Build history of the part. All positions in model axes, mm. A direction names the side the tool comes from. Round coordinates to 2 decimals unless told otherwise and drop trailing zeros. Write each loop counter-clockwise with the first axis right and the second up, starting at its lowest first coordinate (ties: lowest second). Pieces come first, ordered by that corner, then holes. Notation, with made-up numbers: M 5,21 L 23,21 A4 ccw 23,26 Z; hole C 12,-10 d10. An arc over 180 degrees is marked long. Write item = value, one per line. Start each with the question number.
Q1. Band-saw the part on A-A on x = 0. Write the cut outline in (y, z).
Q2. Drop flat-ended pins along their axis: P1, Ø1.5, axis at y = 0, z = 2.5, coming from the +X side; P2, Ø1, axis at y = -2.5, z = -1.5, coming from the +X side; P3, Ø1.5, axis at x = -0.5, y = -5.5, coming from the +Z side. Give the stop position or say it passes through.
Q3. Tool access for faces 1 (the flat face through (4.96, 2.81, -1.65)), 2 (the cylindrical face through (0, 2, 7)), 3 (the flat face through (0, 5.7, -2)), 4 (the flat face through (0, -5.7, -2)): list every direction of +Z, -Z, +X, -X, +Y, -Y with a clear straight run to the whole face (end or side of a thin tool).
Q4. Band-saw the part on B-B on y = 4. Write the cut outline in (x, z), plus the area to 3 significant figures.
Q5. Probe L1, parallel to Z at x = 5, y = 2.25; L2, parallel to Y at x = 1.5, z = -0.75; L3, parallel to X at y = -0.75, z = 0.5. List the from-to ranges inside material, lowest first.
Q6. Band-saw the part on C-C on z = 0.5. Write the cut outline in (x, y), plus the area to 3 significant figures.
Q7. Band-saw the part on D-D on x = 2.75. Write the cut outline in (y, z), plus the area to 3 significant figures.
```python
from build123d import *

# Parameters (mm, degrees)
SKETCH1_R           = 7.5
SKETCH1_R_2         = 5.6
BOSS_EXTRUDE1_DEPTH = 1
BOSS_EXTRUDE2_DEPTH = 3.35
BOSS_EXTRUDE3_START = 1
SKETCH1_4_R         = 5.6
BOSS_EXTRUDE3_DEPTH = 3
BOSS_EXTRUDE4_DEPTH = 5


with BuildPart() as part:
    # Sketch1 → Boss-Extrude1 (new body)
    with BuildSketch(Plane.XY):
        Circle(SKETCH1_R)
        Polygon((-3.290896534, 5.7), (-6.581793069, 0), (-3.290896534, -5.7), (3.290896534, -5.7), (6.581793069, 0), (3.290896534, 5.7), align=None, mode=Mode.SUBTRACT)
        Circle(SKETCH1_R)
        Circle(SKETCH1_R_2, mode=Mode.SUBTRACT)
        Circle(SKETCH1_R_2)
    extrude(amount=BOSS_EXTRUDE1_DEPTH)

    # Sketch1<3> → Boss-Extrude2 (add)
    with BuildSketch(Plane.XY):
        Polygon((-3.290896534, -5.7), (3.290896534, -5.7), (6.581793069, 0), (3.290896534, 5.7), (-3.290896534, 5.7), (-6.581793069, 0), align=None)
    extrude(amount=-BOSS_EXTRUDE2_DEPTH)

    # Sketch1<4> → Boss-Extrude3 (add)
    with BuildSketch(Plane.XY.offset(BOSS_EXTRUDE3_START)):
        Circle(SKETCH1_4_R)
    extrude(amount=BOSS_EXTRUDE3_DEPTH)

    # Sketch2 → Boss-Extrude4 (add, symmetric)
    with BuildSketch(Plane.XY.offset(4)):
        with BuildLine():
            Line((-1.833030278, -0.8), (1.833030278, -0.8))
            ThreePointArc((1.833030278, -0.8), (0, 2), (-1.833030278, -0.8))
        make_face()
    extrude(amount=BOSS_EXTRUDE4_DEPTH, both=True)


solid = part.part
```
Conclusion:
q1.outline = M -7.5,0 L -5.7,0 L -5.7,-3.35 L 5.7,-3.35 L 5.7,0 L 7.5,0 L 7.5,1 L 5.6,1 L 5.6,4 L 2,4 L 2,9 L -0.8,9 L -0.8,4 L -5.6,4 L -5.6,1 L -7.5,1 Z
q2.P1 = 5.6
q2.P2 = 5.43
q2.P3 = 4
q3.face_1 = -Z, +X, +Y
q3.face_2 = +Z
q3.face_3 = -Z, +X, -X, +Y
q3.face_4 = -Z, +X, -X, -Y
q4.outline = M -6.34,0 L -4.27,0 L -4.27,-3.35 L 4.27,-3.35 L 4.27,0 L 6.34,0 L 6.34,1 L 3.92,1 L 3.92,4 L -3.92,4 L -3.92,1 L -6.34,1 Z
q4.area = 64.8 mm^2
q5.L1 = -3.35 to 4
q5.L2 = -5.7 to 5.7
q5.L3 = -7.46 to 7.46
q6.outline = C 0,0 d15
q6.area = 177 mm^2
q7.outline = M -6.98,0 L -5.7,0 L -5.7,-3.35 L 5.7,-3.35 L 5.7,0 L 6.98,0 L 6.98,1 L 4.88,1 L 4.88,4 L -4.88,4 L -4.88,1 L -6.98,1 Z
q7.area = 81.4 mm^2
